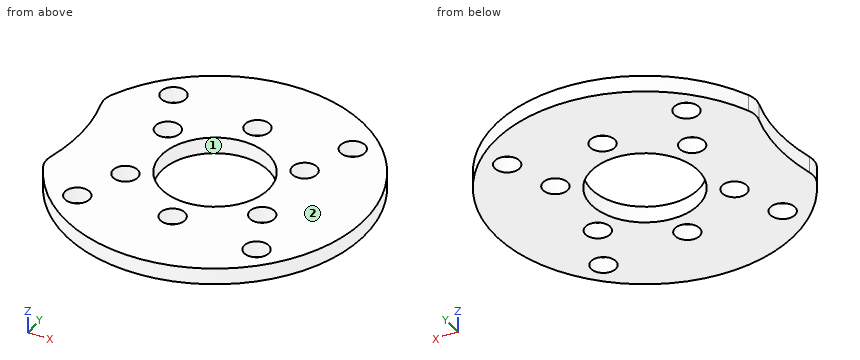
from build123d import *

# Parameters (mm, degrees)
SKETCH_1_R               = 18.25
SKETCH_1_R_2             = 6.55
EXTRUDE_1_DEPTH          = 2
SKETCH_2_R               = 22
CUT_EXTRUDE_1_DEPTH      = 2
SKETCH_3_R               = 1.505
CUT_EXTRUDE_2_DEPTH      = 2
PATTERN_CIRCULAR_1_COUNT = 2
SKETCH_4_R               = 1.505
CUT_EXTRUDE_3_DEPTH      = 2
FILLET_1_R               = 3


with BuildPart() as part:
    # 草图1 → 凸台-拉伸1 (new body)
    with BuildSketch(Plane.XY):
        Circle(SKETCH_1_R)
        Circle(SKETCH_1_R_2, mode=Mode.SUBTRACT)
    extrude(amount=EXTRUDE_1_DEPTH)

    # 草图2 → 切除-拉伸1 (cut)
    with BuildSketch(Plane.XY.offset(2)):
        with Locations((-38, 0)):
            Circle(SKETCH_2_R)
    extrude(amount=-CUT_EXTRUDE_1_DEPTH, mode=Mode.SUBTRACT)

    # 草图3 → 切除-拉伸2 (cut)
    with BuildSketch(Plane.XY.offset(2)):
        with Locations((0, 9.5)):
            Circle(SKETCH_3_R)
        with Locations((8.227241336, -4.75)):
            Circle(SKETCH_3_R)
        with Locations((-8.227241336, -4.75)):
            Circle(SKETCH_3_R)
    cut_extrude_2 = extrude(amount=-CUT_EXTRUDE_2_DEPTH, mode=Mode.SUBTRACT)

    # 阵列(圆周)1: 切除-拉伸2 ×2 about axis
    pattern_circular_1_axis = Axis((0, 0, 0), (0, 0, 1))
    for i in range(1, PATTERN_CIRCULAR_1_COUNT):
        add(cut_extrude_2.rotate(pattern_circular_1_axis, i * 360 / PATTERN_CIRCULAR_1_COUNT), mode=Mode.SUBTRACT)

    # 草图4 → 切除-拉伸3 (cut)
    with BuildSketch(Plane.XY.offset(2)):
        with Locations((-10.783378413, 10.783378413)):
            Circle(SKETCH_4_R)
        with Locations((10.783378413, 10.783378413)):
            Circle(SKETCH_4_R)
        with Locations((10.783378413, -10.783378413)):
            Circle(SKETCH_4_R)
        with Locations((-10.783378413, -10.783378413)):
            Circle(SKETCH_4_R)
    extrude(amount=-CUT_EXTRUDE_3_DEPTH, mode=Mode.SUBTRACT)

    # 圆角1
    fillet_1_edges = [part.edges().sort_by_distance(p)[0] for p in [
        (-17.013980263, -6.60204329, 1),
        (-17.013980263, 6.60204329, 1),
    ]]
    fillet(fillet_1_edges, radius=FILLET_1_R)


solid = part.part
The listing builds one solid part. Answer for the finished solid, in the listing's coordinates (mm). Face numbers are marked on the shaded views. Coordinates: 2 decimals unless noted, no trailing zeros. Write each loop counter-clockwise with the first axis right and the second up, starting at its lowest first coordinate (ties: lowest second). Pieces come first, ordered by that corner, then holes. Notation, with made-up numbers: M 26,-17 L 62,-17 A20 cw 62,6 Z; hole C 10.5,45.25 d8. An arc over 180 degrees is marked long. Use one line per item in the form item = value.
Item 1: Find section A-A, the plane y = 0. Give the vertices of the cut face in (x, z).
Model answer:
outline = M -16,0 L -6.55,0 L -6.55,2 L -16,2 Z; M 6.55,0 L 18.25,0 L 18.25,2 L 6.55,2 Z
Item 2: Find the intervals of material crossed by probe 1 along Y at (x, z) = (0, 0.15) (3 decimals); probe 2 along X at (y, z) = (10, 1); probe 3 along Y at (x, z) = (-7.5, 1.5), in increasing order.
Model answer:
probe_1 = -18.25 to -11.005, -7.995 to -6.55, 6.55 to 7.995, 11.005 to 18.25
probe_2 = -15.27 to -12.07, -9.5 to -1.42, 1.42 to 9.5, 12.07 to 15.27
probe_3 = -16.64 to -6.07, -3.43 to 3.43, 6.07 to 16.64
Item 3: Find section C-C, the plane y = -4.75. Give the vertices of the cut face in (x, z), plus the area to 3 significant figures.
Model answer:
outline = M -16.52,0 L -9.73,0 L -9.73,2 L -16.52,2 Z; M -6.72,0 L -4.51,0 L -4.51,2 L -6.72,2 Z; M 4.51,0 L 6.72,0 L 6.72,2 L 4.51,2 Z; M 9.73,0 L 17.62,0 L 17.62,2 L 9.73,2 Z
area = 38.2 mm2
Item 4: Find section D-D, the plane x = -8. Give the vertices of the cut face in (y, z).
Model answer:
outline = M -16.4,0 L -6.24,0 L -6.24,2 L -16.4,2 Z; M -3.26,0 L 3.26,0 L 3.26,2 L -3.26,2 Z; M 6.24,0 L 16.4,0 L 16.4,2 L 6.24,2 Z
Item 5: Find section B-B, the plane x = 5.5. Give the vertices of the cut face in (y, z).
Model answer:
outline = M -17.4,0 L -3.56,0 L -3.56,2 L -17.4,2 Z; M 3.56,0 L 17.4,0 L 17.4,2 L 3.56,2 Z
Item 6: The mould has two halves that part along Y. Classify the marked faces 1 and 2: released by +Y, released by -Y, zero draft, split by the parting line, or undercut.
Model answer:
face_1 = undercut
face_2 = zero draft
Item 7: Given P1, Ø2.5, axis at x = -10.78, y = -10.78, coming from the -Z side, flat-ended and moving along its own axis, determine where the tip first touches the part or whether it passes through.
Model answer:
P1 = through
